Read the model definition and answer for the solid it produces. Units are mm, in the model's axes. Face numbers are marked on the shaded views. A direction names the side the tool comes from. Round coordinates to 2 decimals unless told otherwise and drop trailing zeros. Order: outer loops, then holes, each group sorted by start corner. A loop starts at its lowest first (then second) coordinate and runs counter-clockwise, first axis right, second up. Notation, with made-up numbers: (32, -24.5) - (52, -24.5) arc R23 ccw to (52, -5.5) - close; hole circle Ø2 at (47, 18). An arc over 180 degrees is marked (long way). Answer as a JSON object with one key per item and string values. Group by question number.
Q1. A cutting plane is placed at C-C on y = 38. Determine the outline of the cut face in (x, z), and give its area (3 significant figures).
Q2. The mould has two halves that part along Y. Classify the marked faces 3, 4, 5 and 6: pulls with the +Y half, pulls with the -Y half, needs draft (parallel to the pull), parting line crosses it, or undercut.
Q3. A cutting plane is placed at A-A on y = 20. Determine the outline of the cut face in (x, z), and give its area (3 significant figures).
Q4. A tool of negligible diameter and unlimited length cuts with its end or side. For the marked faces 1 and 2, from which of +Z, -Z, +X, -X, +Y, -Y can it reach the whole face along a straight path? Write none if from no direction.
Q5. A cutting plane is placed at B-B on z = 20. Determine the outline of the cut face in (x, y).
Q6. Consider line 1 (Y direction, x = 2.8, z = 20); line 2 (Y direction, x = 2.05, z = 18); line 3 (Z direction, x = 4.55, y = 33). Determine where each line is inside the solid, lowest interval first.
Q7. Given pin 1 Ø1.5 at (x, y) = (1.5, 1) entering from -Z; pin 2 Ø1.5 at (x, y) = (0.5, 19.5) entering from +Z; pin 3 Ø3 at (x, z) = (2, 24.5) entering from -Y, each flat-ended and moving along its own axis, determine where each tip first touches the part or whether it passes through.
Q8. A cutting plane is placed at D-D on z = 29. Determine the outline of the cut face in (x, y), and give its area (3 significant figures).
```python
from build123d import *

# Parameters (mm, degrees)
SKETCH_1_R          = 5.2
EXTRUDE_1_DEPTH     = 5
SKETCH_2_W          = 5
SKETCH_2_H          = 10
CUT_EXTRUDE_1_DEPTH = 62.23724357


with BuildPart() as part:
    # Эскиз1 → Бобышка-Вытянуть1 (new body)
    with BuildSketch(Plane(origin=(0, 0, 0), x_dir=(0, 0, -1), z_dir=(1, 0, 0))):
        with BuildLine():
            Line((0, 0), (-5, 0))
            Line((-5, 0), (-5, -10))
            ThreePointArc((-5, -10), (-35, 20), (-5, 50))
            Line((-5, 50), (-5, 40))
            Line((-5, 40), (0, 40))
            Line((0, 40), (0, 0))
        make_face()
        with Locations((-20, 20)):
            Circle(SKETCH_1_R, mode=Mode.SUBTRACT)
    extrude(amount=EXTRUDE_1_DEPTH)

    # Эскиз2 → Вырез-Вытянуть1 (cut, through all)
    with BuildSketch(Plane(origin=(5, 0, 0), x_dir=(0, 0, -1), z_dir=(1, 0, 0))):
        with Locations((-2.5, 35)):
            Rectangle(SKETCH_2_W, SKETCH_2_H)
        with Locations((-2.5, 5)):
            Rectangle(SKETCH_2_W, SKETCH_2_H)
    extrude(amount=-CUT_EXTRUDE_1_DEPTH, mode=Mode.SUBTRACT)


solid = part.part
```
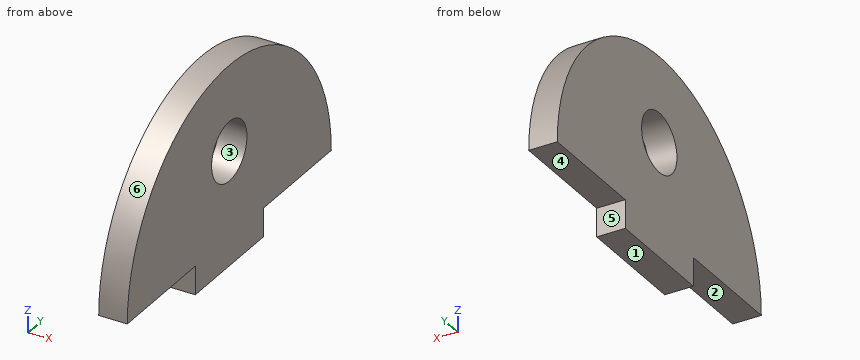
Result set:
{
 "1": {"outline": "(0, 5) - (5, 5) - (5, 29) - (0, 29) - close", "area": "120 mm²"},
 "2": {"face 3": "undercut", "face 4": "needs draft", "face 5": "pulls with the +Y half", "face 6": "parting line crosses it"},
 "3": {"outline": "(0, 0) - (5, 0) - (5, 14.8) - (0, 14.8) - close; (0, 25.2) - (5, 25.2) - (5, 35) - (0, 35) - close", "area": "123 mm²"},
 "4": {"face 1": "-Z, +X, -X, +Y, -Y", "face 2": "-Z, +X, -X, -Y"},
 "5": {"outline": "(0, -5.98) - (5, -5.98) - (5, 14.8) - (0, 14.8) - close; (0, 25.2) - (5, 25.2) - (5, 45.98) - (0, 45.98) - close"},
 "6": {"line 1": "y = -5.98 to 14.8, 25.2 to 45.98", "line 2": "y = -7.04 to 15.2, 24.8 to 47.04", "line 3": "z = 5 to 32.04"},
 "7": {"pin 1": "stops at z = 5", "pin 2": "stops at z = 35", "pin 3": "stops at y = -4"},
 "8": {"outline": "(0, 2) - (5, 2) - (5, 38) - (0, 38) - close", "area": "180 mm²"}
}
